Here's the drawing with two shaded views (mm, measured from the low corner). I have some questions. Round coordinates to 2 decimals unless told otherwise and drop trailing zeros. Order: outer loops, then holes, each group sorted by start corner. A loop starts at its lowest first (then second) coordinate and runs counter-clockwise, first axis right, second up.
Q1. If we section it at C-C (x = 24): Please give me the cut outline in (y, z), plus the area to 3 significant figures.
Q2. If we section it at B-B (y = 4.5): Please give me the cut outline in (x, z), plus the area to 3 significant figures.
Q3. If we section it at A-A (z = 4.4): Please give me the cut outline in (x, y).
Q4. If I drill on line 1 (Y direction, x = 23, z = 4.9); line 2 (Z direction, x = 39.5, y = 4.75), over which ranges is the centre line in solid material (lowest first)?
Q5. Will this pin go through, and if not, where does the flat tip stop? P1, Ø2, axis at x = 18, y = 7, coming from the +Z side.
Q6. If we section it at D-D (z = 0.7): Please give me the cut outline in (x, y).
Q7. We'd pull the mould along X, two halves only. Please class the marked faces 1 and 2: pulls with the +X half, pulls with the -X half, needs draft (parallel to the pull), parting line crosses it, or undercut.
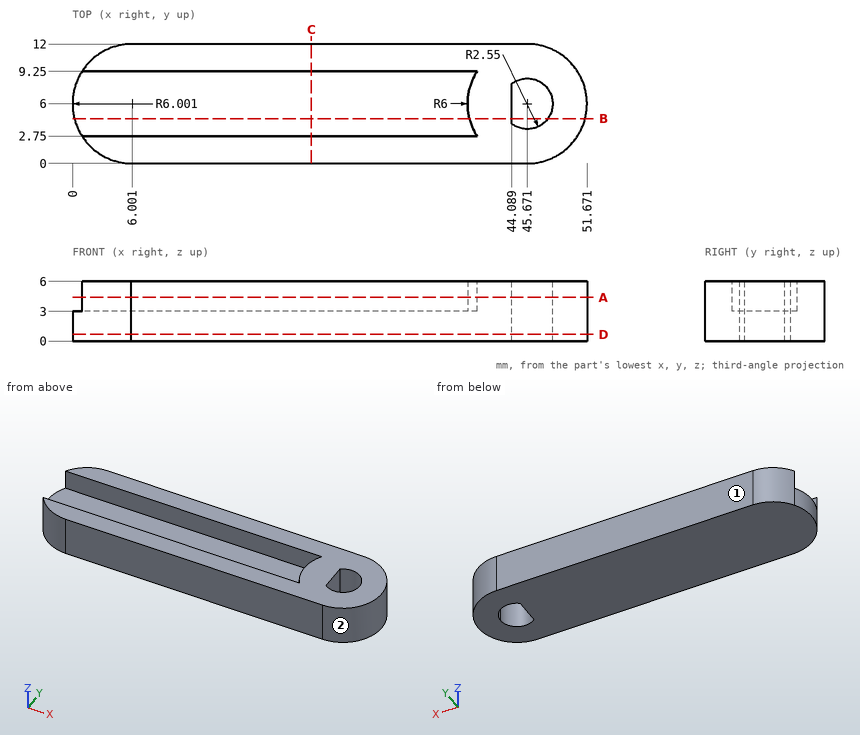
Solution:
1. outline: (0, 0) - (12, 0) - (12, 6) - (9.25, 6) - (9.25, 3) - (2.75, 3) - (2.75, 6) - (0, 6) - close
1. area: 52.5 mm2
2. outline: (0.19, 0) - (44.09, 0) - (44.09, 6) - (39.86, 6) - (39.86, 3) - (0.19, 3) - close; (47.73, 0) - (51.48, 0) - (51.48, 6) - (47.73, 6) - close
2. area: 167 mm2
3. outline: (0.96, 2.75) arc R6 ccw to (5.92, 0) - (45.67, 0) arc R6 ccw to (45.67, 12) - (5.92, 12) arc R6 ccw to (0.96, 9.25) - (40.63, 9.25) arc R6 ccw to (40.63, 2.75) - close; hole (44.09, 4) arc R2.55 ccw (long way) to (44.09, 8) - close
4. line 1: y = 0 to 2.75, 9.25 to 12
4. line 2: z = 0 to 3
5. P1: stops at z = 3
6. outline: (5.92, 0) - (45.67, 0) arc R6 ccw to (45.67, 12) - (5.92, 12) arc R6 ccw to start; hole (44.09, 4) arc R2.55 ccw (long way) to (44.09, 8) - close
7. face 1: needs draft
7. face 2: pulls with the +X half
